```python
from build123d import *

# Parameters (mm, degrees)
SKETCH1_R           = 1.5
BOSS_EXTRUDE1_DEPTH = 4.5
FILLET1_RADIUS      = 4.5
FILLET1_LENGTH      = 3.9
CUT_EXTRUDE1_REACH  = 37.558
SKETCH3_R           = 1.5
CHAMFER1_SIZE       = 0.6
CHAMFER2_SIZE       = 0.4


with BuildPart() as part:
    # Sketch1 → Boss-Extrude1 (new, symmetric)
    with BuildSketch(Plane.XY):
        with BuildLine():
            Line((-13.05, 0), (-13.05, 8.691684344))
            ThreePointArc((-13.05, 8.691684344), (-12.675231148, 10.382157391), (-11.621150439, 11.755862116))
            Line((-11.621150439, 11.755862116), (-9.365773473, 13.648348096))
            ThreePointArc((-9.365773473, 13.648348096), (-8.36559922, 14.262761606), (-7.230139126, 14.560390355))
            ThreePointArc((-7.230139126, 14.560390355), (-3.689610404, 15.637001914), (-0.783040807, 17.927479867))
            ThreePointArc((-0.783040807, 17.927479867), (0.108053117, 18.688045586), (1.181284206, 19.15781534))
            ThreePointArc((1.181284206, 19.15781534), (2.248897725, 27.397750508), (-4.350434235, 22.349468831))
            ThreePointArc((-4.350434235, 22.349468831), (-4.87363913, 19.752292641), (-7.250723724, 18.582448052))
            Line((-7.250723724, 18.582448052), (-8.250559688, 18.582448052))
            ThreePointArc((-8.250559688, 18.582448052), (-9.618640261, 18.341218535), (-10.821710127, 17.646625825))
            Line((-10.821710127, 17.646625825), (-15.521150439, 13.703327192))
            ThreePointArc((-15.521150439, 13.703327192), (-16.575231148, 12.329622467), (-16.95, 10.63914942))
            Line((-16.95, 10.63914942), (-16.95, 0))
            Line((-16.95, 0), (-13.05, 0))
        make_face()
        with Locations((0, 23.5)):
            Circle(SKETCH1_R, mode=Mode.SUBTRACT)
    extrude(amount=BOSS_EXTRUDE1_DEPTH, both=True)

    # Fillet1: full round fillet: the end face becomes a half cylinder, R = half its width
    fillet1_face = Plane((-15, 0, 0), x_dir=(-1, 0, 0), z_dir=(0, -1, 0))  # on the end face: x along it, z out of the body
    fillet1_slab = fillet1_face.offset(-FILLET1_RADIUS / 2) * Box(FILLET1_LENGTH, 2 * FILLET1_RADIUS, FILLET1_RADIUS, mode=Mode.PRIVATE)  # the body's end, R deep
    fillet1_round = Plane((-15, 4.5, 0), x_dir=(0, -1, 0), z_dir=(-1, 0, 0)) * Cylinder(FILLET1_RADIUS, FILLET1_LENGTH, mode=Mode.PRIVATE)  # its axis R under the face
    add(fillet1_slab - fillet1_round, mode=Mode.SUBTRACT)

    # Sketch3 → Cut-Extrude1 (cut, up to next)
    with BuildSketch(Plane.ZY.offset(16.95), mode=Mode.PRIVATE) as cut_extrude1_sk1:
        with Locations((0, 4.5)):
            Circle(SKETCH3_R)
    cut_extrude1_tool1 = extrude(cut_extrude1_sk1.sketch, amount=-CUT_EXTRUDE1_REACH, mode=Mode.PRIVATE) & part.part
    add(cut_extrude1_tool1.solids().sort_by_distance((-16.95, 4.5, 0))[0], mode=Mode.SUBTRACT)

    # Chamfer1
    chamfer1_edges = [part.edges().sort_by_distance(p)[0] for p in [
        (-13.171430283, 15.674976508, -4.5),
        (-9.618640261, 18.341218535, -4.5),
        (-7.750641706, 18.582448052, -4.5),
        (-4.87363913, 19.752292641, -4.5),
        (2.248897725, 27.397750508, -4.5),
        (0.108053117, 18.688045586, -4.5),
        (-3.689610404, 15.637001914, -4.5),
        (-8.36559922, 14.262761606, -4.5),
        (-10.493461956, 12.702105106, -4.5),
        (-12.675231148, 10.382157391, 4.5),
        (-12.675231148, 10.382157391, -4.5),
        (-16.95, 7.56957471, -4.5),
        (-16.575231148, 12.329622467, -4.5),
        (-10.493461956, 12.702105106, 4.5),
        (-8.36559922, 14.262761606, 4.5),
        (-3.689610404, 15.637001914, 4.5),
        (0.108053117, 18.688045586, 4.5),
        (2.248897725, 27.397750508, 4.5),
        (-4.87363913, 19.752292641, 4.5),
        (-7.750641706, 18.582448052, 4.5),
        (-16.575231148, 12.329622467, 4.5),
        (-9.618640261, 18.341218535, 4.5),
        (-13.171430283, 15.674976508, 4.5),
        (-13.05, 6.595842172, -4.5),
        (-13.05, 6.595842172, 4.5),
        (-13.05, 0, 0),
        (-16.95, 0, 0),
        (-16.95, 7.56957471, 4.5),
    ]]
    chamfer(chamfer1_edges, length=CHAMFER1_SIZE)

    # Chamfer2
    chamfer2_edges = [part.edges().sort_by_distance(p)[0] for p in [
        (-1.5, 23.5, -4.5),
        (-1.5, 23.5, 4.5),
        (-16.95, 4.5, -1.5),
        (-13.05, 4.5, -1.5),
    ]]
    chamfer(chamfer2_edges, length=CHAMFER2_SIZE)


solid = part.part
```
CAD build for the part. Positions are in the model's coordinates, mm. A direction names the side the tool comes from. Give positions to 0.01 mm unless a question says otherwise; leave off trailing zeros. Loops run counter-clockwise (first coordinate to the right, second up) from the corner with the lowest first, then second, coordinate; pieces in that order, holes last. Notation, with made-up numbers: M -22,-7.5 L 18,-7.5 A22 ccw 18,8.5 Z; hole C 68.25,42 d6. An arc over 180 degrees is marked long. Use one line per item in the form item = value.
Item 1: Which spindle directions (+Z, -Z, +X, -X, +Y, -Y) get a long thin tool onto all of the face, cutting with end or side? Do faces 1 (the face through (-8, 18.582, 0)), 2 (the face through (-7, 17, -4.5)). Say none if no direction does.
Determined:
face_1 = +Z, -Z, -X, +Y
face_2 = -Z, +X, -X, +Y, -Y
Item 2: Slice it at C-C (x = -14.25). List the corners of the cut face in (y, z), plus the area to 3 significant figures.
Determined:
outline = M 4.5,-4.5 L 13.99,-4.5 L 14.77,-3.9 L 14.77,3.9 L 13.99,4.5 L 4.5,4.5 A4.5 ccw Z; hole C 4.5,0 d3
area = 117 mm2
Item 3: Drill centre lines: probe 1 along Y at (x, z) = (-14.5, 0); probe 2 along X at (y, z) = (2.5, -2.25); probe 3 along Y at (x, z) = (-14.95, 0). Where is each one in solid material? Low to high. Write a range as from..to.
Determined:
probe_1 = 0..3, 6..14.56
probe_2 = -16.95..-13.05
probe_3 = 0..3, 6..14.18
Item 4: Slice it at B-B (z = 0). List the corners of the cut face in (x, y).
Determined:
outline = M -16.95,0.6 L -16.35,0 L -13.65,0 L -13.05,0.6 L -13.05,2.6 L -13.45,3 L -16.55,3 L -16.95,2.6 Z; M -16.95,6.4 L -16.55,6 L -13.45,6 L -13.05,6.4 L -13.05,8.69 A4 cw -11.62,11.76 L -9.37,13.65 A4 cw -7.23,14.56 A10 ccw -0.78,17.93 A4 cw 1.18,19.16 A4.5 ccw long -4.35,22.35 A3 cw -7.25,18.58 L -8.25,18.58 A4 ccw -10.82,17.65 L -15.52,13.7 A4 ccw -16.95,10.64 Z; hole C 0,23.5 d3
Item 5: Slice it at A-A (y = 23.5). List the corners of the cut face in (x, z), plus the area to 3 significant figures.
Determined:
outline = M -4.5,-3.9 L -3.9,-4.5 L -1.9,-4.5 L -1.5,-4.1 L -1.5,4.1 L -1.9,4.5 L -3.9,4.5 L -4.5,3.9 Z; M 1.5,-4.1 L 1.9,-4.5 L 3.9,-4.5 L 4.5,-3.9 L 4.5,3.9 L 3.9,4.5 L 1.9,4.5 L 1.5,4.1 Z
area = 53.0 mm2
Item 6: Two-plate mould, pull along Y, no slides. Class faces 3 (the face through (-15.02, 4.57, -1.5)), 4 (the face through (-16.79, 0.44, -0.09)), 5 (the face through (-16.24, 12.2, -4.26)): pulls with the +Y half, pulls with the -Y half, needs draft (parallel to the pull), parting line crosses it, or undercut.
Determined:
face_3 = undercut
face_4 = pulls with the -Y half
face_5 = pulls with the +Y half
Item 7: Flat gauge pins, fed straight in: pin 1 (1.1 mm diameter, centred on x = -8, z = 1, fed in from +Y); pin 2 (1 mm diameter, centred on y = 20.5, z = 0.5, fed in from +X); pin 3 (4 mm diameter, centred on y = 21.5, z = -1.5, fed in from -X); pin 4 (10 mm diameter, centred on x = -8, y = 3.5, fed in from +Z). Where does each tip first touch, or does it go through?
Determined:
pin_1 = 18.58
pin_2 = 3.74
pin_3 = -5.09
pin_4 = through
